```python
from build123d import *

# Parameters (mm, degrees)
F0_W     = 25
F0_H     = 11.5
F0_R     = 1.7
F1_DEPTH = 3
F0_H_2   = 15
F0_R_2   = 4.6
F0_R_3   = 2.7
F2_DEPTH = 6
F3_DEPTH = 2
F4_SIZE  = 2.99999
F5_START = 2
F5_DEPTH = 0.3


# Not quite as in the source:
# - a fillet or chamfer is up to 0.001 mm smaller than in the source, because OpenCascade refuses the exact size


with BuildPart() as f1:
    # F0 (on Top) → F1 (new body)
    with BuildSketch(Plane.XY):
        with Locations((0, 13.25)):
            Rectangle(F0_W, F0_H)
        with Locations((0, 14)):
            Circle(F0_R, mode=Mode.SUBTRACT)
    extrude(amount=F1_DEPTH)



with BuildPart() as f1b:
    # F0 (on Top) → F1, piece 2 (new body)
    with BuildSketch(Plane.XY):
        with Locations((0, -13.25)):
            Rectangle(F0_W, F0_H)
        with Locations((0, -14)):
            Circle(F0_R, mode=Mode.SUBTRACT)
    extrude(amount=F1_DEPTH)


with BuildPart() as f1_1:
    add(f1.part)

    add(f1b.part)  # F2 merges F1b
    # F0 (on Top) → F2 (join)
    with BuildSketch(Plane.XY):
        Rectangle(F0_W, F0_H_2)
        Circle(F0_R_2, mode=Mode.SUBTRACT)
        Circle(F0_R_2)
        Circle(F0_R_3, mode=Mode.SUBTRACT)
    extrude(amount=F2_DEPTH)

    # F0 (on Top) → F3 (cut)
    with BuildSketch(Plane.XY):
        Circle(F0_R_2)
        Circle(F0_R_3, mode=Mode.SUBTRACT)
    extrude(amount=F3_DEPTH, mode=Mode.SUBTRACT)

    # F4 (size 3 in the source; OpenCascade refuses exactly that, so slightly less here)
    f4_edges = [f1_1.edges().sort_by_distance(p)[0] for p in [
        (0, 7.5, 3),
        (0, -7.5, 3),
        (12.5, -19, 1.5),
        (-12.5, -19, 1.5),
        (12.5, 19, 1.5),
        (-12.5, 19, 1.5),
    ]]
    chamfer(f4_edges, length=F4_SIZE)

    # F0 (on Top) → F5 (join)
    with BuildSketch(Plane.XY.offset(F5_START)):
        Circle(F0_R_3)
    extrude(amount=F5_DEPTH)


solid = f1_1.part
```
The listing builds one solid part. Answer for the finished solid, in the listing's coordinates (mm). A direction names the side the tool comes from. Round coordinates to 2 decimals unless told otherwise and drop trailing zeros. Loops run counter-clockwise (first coordinate to the right, second up) from the corner with the lowest first, then second, coordinate; pieces in that order, holes last.
1) For a pull along X with two mould halves and no side action, classify faces 6 (the face through (0, 0, 2)), 7 (the face through (12.5, 0, 2)), 8 (the face through (0, 19, 1)) as released by +X, released by -X, zero draft, split by the parting line, or undercut.
Outcome:
face 6: undercut
face 7: released by +X
face 8: zero draft
2) Consider line 1 (Y direction, x = 0, z = 2.35); line 2 (Y direction, x = 0, z = 1.65); line 3 (Z direction, x = -7.25, y = 14.5). Determine where each line is inside the solid, lowest interval first.
Outcome:
line 1: y = -19 to -15.7, -12.3 to -2.7, 2.7 to 12.3, 15.7 to 19
line 2: y = -19 to -15.7, -12.3 to -4.6, 4.6 to 12.3, 15.7 to 19
line 3: z = 0 to 3
3) A cutting plane is placed at B-B on y = 14. Determine the outline of the cut face in (x, z), plus the area to 3 significant figures.
Outcome:
outline: (-12.5, 0) - (-1.7, 0) - (-1.7, 3) - (-12.5, 3) - close; (1.7, 0) - (12.5, 0) - (12.5, 3) - (1.7, 3) - close
area: 64.8 mm2
4) A cutting plane is placed at C-C on z = 1.4. Determine the outline of the cut face in (x, y).
Outcome:
outline: (-12.5, -16) - (-9.5, -19) - (9.5, -19) - (12.5, -16) - (12.5, 16) - (9.5, 19) - (-9.5, 19) - (-12.5, 16) - close; hole circle Ø9.2 at (0, 0); hole circle Ø3.4 at (0, -14); hole circle Ø3.4 at (0, 14)
5) For faces 1 (the face through (-11, -17.5, 1.5)), 2 (the face through (-3.65, -2.8, 0.99)), 3 (the face through (0, -17, 3)), 4 (the face through (0, 16, 3)), 5 (the face through (-0.585, -2.636, 4.124)), determine the directions among +Z, -Z, +X, -X, +Y, -Y from which every point of the face is accessible in a straight line to the end or side of a thin tool.
Outcome:
face 1: +Z, -Z, -X, -Y
face 2: -Z
face 3: +Z, +X, -X, -Y
face 4: +Z, +X, -X, +Y
face 5: +Z
6) A cutting plane is placed at A-A on x = 0. Give the number of separate pieces and of enclosed holes in the cut face, plus the area to 3 significant figures.
Outcome:
separate pieces: 3
enclosed holes: 0
area: 109 mm2
7) Given P1, Ø3, axis at x = 9, y = -6, coming from the -Z side; P2, Ø3, axis at x = 2, y = -0.5, coming from the -Z side; P3, Ø5.5, axis at x = 0, y = 14, coming from the +Z side, each flat-ended and moving along its own axis, determine where each tip first touches the part or whether it passes through.
Outcome:
P1: stops at z = 0
P2: stops at z = 2
P3: stops at z = 3
